from build123d import *

# Parameters (mm, degrees)
FILLET1_R = 0.4


# Read off the part's stored shape, not the designer's step: Revolve1
with BuildPart() as part:
    # Revolve1 outline → Revolve1 (revolve)
    with BuildSketch(Plane.XY):
        Polygon((15.445079495, 5), (10.445079495, 0), (12, 0), (17, 5), (12, 8), (10.445079495, 8), align=None)
    revolve(axis=Axis((0, 0, 0), (0, 1, 0)))

    # Fillet1
    fillet1_edges = [part.edges().sort_by_distance(p)[0] for p in [
        (-15.445079495, 5, 0),
    ]]
    fillet(fillet1_edges, radius=FILLET1_R)


solid = part.part
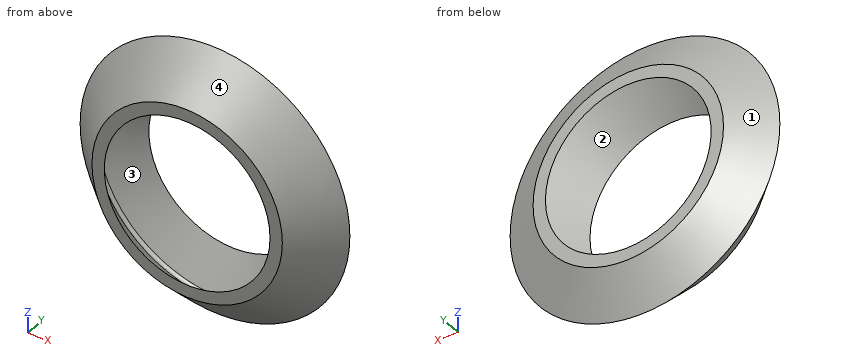
Work out the finished part from the listing and answer in its coordinate system (mm). Face numbers are marked on the shaded views. A direction names the side the tool comes from. Coordinates: 2 decimals unless noted, no trailing zeros. Write each loop counter-clockwise with the first axis right and the second up, starting at its lowest first coordinate (ties: lowest second). Pieces come first, ordered by that corner, then holes. Notation, with made-up numbers: M 43,46 L 88,46 A15 ccw 88,59 Z; hole C -21.75,10 d10. An arc over 180 degrees is marked long. Use one line per item in the form item = value. Start each with the question number.
1. The mould has two halves that part along Z. Classify the marked faces 3 and 4: released by +Z, released by -Z, zero draft, split by the parting line, or undercut.
2. This flat-tipped pin is pushed along its axis until it touches: P1, Ø1, axis at x = 10.5, z = 4, coming from the -Y side. Where does it stop, or does it pass through?
3. Straight lines are drawn through the part: probe 1 along X at (y, z) = (1.5, 7.5); probe 2 along Z at (x, y) = (5.5, 7); probe 3 along X at (y, z) = (2, -1.5). For each, find the intervals that lie inside material, in ascending order. Write a range as from..to.
4. A tool of negligible diameter and unlimited length cuts with its end or side. For the marked faces 1 and 2, from which of +Z, -Z, +X, -X, +Y, -Y can it reach the whole face along a straight path? Write none if from no direction.
5. The part is cut by section B-B (y = 6.5). Give the vertices of the cut face in (x, z).
6. The part is cut by section A-A (y = 1.25). Give the vertices of the cut face in (x, z), plus the area to 3 significant figures.
Evaluation:
q1.face_3 = undercut
q1.face_4 = split by the parting line
q2.P1 = 0
q3.probe_1 = -11.22..-9.3, 9.3..11.22
q3.probe_2 = -12.51..-10.79, 10.79..12.51
q3.probe_3 = -13.92..-12.35, 12.35..13.92
q4.face_1 = +Y
q4.face_2 = none
q5.outline = C 0,0 d29; hole C 0,0 d25.89
q6.outline = C 0,0 d26.5; hole C 0,0 d23.39
q6.area = 122 mm^2
